```python
from build123d import *

# Parameters (mm, degrees)
SKETCH_1_W          = 270
SKETCH_1_H          = 136
EXTRUDE_1_DEPTH     = 278
SKETCH_2_W          = 266
SKETCH_2_H          = 274
CUT_EXTRUDE_1_DEPTH = 134
CUT_EXTRUDE_2_REACH = 318.438
SKETCH_3_W          = 100
SKETCH_3_H          = 40
CUT_EXTRUDE_3_REACH = 318.438
SKETCH_4_W          = 1
SKETCH_4_H          = 4


with BuildPart() as part:
    # 草图1 → 凸台-拉伸1 (new body)
    with BuildSketch(Plane(origin=(0, 0, 0), x_dir=(1, 0, 0), z_dir=(0, 1, 0))):
        Rectangle(SKETCH_1_W, SKETCH_1_H)
    extrude(amount=EXTRUDE_1_DEPTH)

    # 草图2 → 切除-拉伸1 (cut)
    with BuildSketch(Plane(origin=(0, 0, -68), x_dir=(-1, 0, 0), z_dir=(0, 0, -1))):
        with Locations((0, 139)):
            Rectangle(SKETCH_2_W, SKETCH_2_H)
    extrude(amount=-CUT_EXTRUDE_1_DEPTH, mode=Mode.SUBTRACT)

    # 草图3 → 切除-拉伸2 (cut, up to next)
    with BuildSketch(Plane(origin=(0, 278, 0), x_dir=(1, 0, 0), z_dir=(0, 1, 0)), mode=Mode.PRIVATE) as cut_extrude_2_sk1:
        with Locations((0, 48)):
            Rectangle(SKETCH_3_W, SKETCH_3_H)
    cut_extrude_2_tool1 = extrude(cut_extrude_2_sk1.sketch, amount=-CUT_EXTRUDE_2_REACH, mode=Mode.PRIVATE) & part.part
    add(cut_extrude_2_tool1.solids().sort_by_distance((0, 278, -48))[0], mode=Mode.SUBTRACT)

    # 草图4 → 切除-拉伸3 (cut, up to next)
    with BuildSketch(Plane.XZ, mode=Mode.PRIVATE) as cut_extrude_3_sk1:
        with Locations((-134.5, 42)):
            Rectangle(SKETCH_4_W, SKETCH_4_H)
    cut_extrude_3_tool1 = extrude(cut_extrude_3_sk1.sketch, amount=-CUT_EXTRUDE_3_REACH, mode=Mode.PRIVATE) & part.part
    # 草图4 → 切除-拉伸3 (cut, up to next)
    with BuildSketch(Plane.XZ, mode=Mode.PRIVATE) as cut_extrude_3_sk2:
        with Locations((-134.5, -42)):
            Rectangle(SKETCH_4_W, SKETCH_4_H)
    cut_extrude_3_tool2 = extrude(cut_extrude_3_sk2.sketch, amount=-CUT_EXTRUDE_3_REACH, mode=Mode.PRIVATE) & part.part
    # 草图4 → 切除-拉伸3 (cut, up to next)
    with BuildSketch(Plane.XZ, mode=Mode.PRIVATE) as cut_extrude_3_sk3:
        with Locations((134.5, -42)):
            Rectangle(SKETCH_4_W, SKETCH_4_H)
    cut_extrude_3_tool3 = extrude(cut_extrude_3_sk3.sketch, amount=-CUT_EXTRUDE_3_REACH, mode=Mode.PRIVATE) & part.part
    # 草图4 → 切除-拉伸3 (cut, up to next)
    with BuildSketch(Plane.XZ, mode=Mode.PRIVATE) as cut_extrude_3_sk4:
        with Locations((134.5, 42)):
            Rectangle(SKETCH_4_W, SKETCH_4_H)
    cut_extrude_3_tool4 = extrude(cut_extrude_3_sk4.sketch, amount=-CUT_EXTRUDE_3_REACH, mode=Mode.PRIVATE) & part.part
    add(cut_extrude_3_tool1.solids().sort_by_distance((-134.5, 0, 42))[0], mode=Mode.SUBTRACT)
    add(cut_extrude_3_tool2.solids().sort_by_distance((-134.5, 0, -42))[0], mode=Mode.SUBTRACT)
    add(cut_extrude_3_tool3.solids().sort_by_distance((134.5, 0, -42))[0], mode=Mode.SUBTRACT)
    add(cut_extrude_3_tool4.solids().sort_by_distance((134.5, 0, 42))[0], mode=Mode.SUBTRACT)


solid = part.part
```
Part model, mm, in its own coordinate system. A direction names the side the tool comes from. Round coordinates to 2 decimals unless told otherwise and drop trailing zeros. Loops run counter-clockwise (first coordinate to the right, second up) from the corner with the lowest first, then second, coordinate; pieces in that order, holes last. Notation, with made-up numbers: (57.25, 77.25) -> (112.25, 77.25) arc R20 cw to (112.25, 103.25) -> close; hole circle Ø2 at (18, -10.75). An arc over 180 degrees is marked (long way). Use a Markdown table: item, result.
1) Cut at D-D, the plane z = -49. List the corners of the cut face in (x, y), and give its area (3 significant figures).
The answers:
| item | result |
|---|---|
| outline | (-135, 0) -> (135, 0) -> (135, 278) -> (50, 278) -> (50, 276) -> (133, 276) -> (133, 2) -> (-133, 2) -> (-133, 276) -> (-50, 276) -> (-50, 278) -> (-135, 278) -> close |
| area | 1,980 mm2 |
2) Probe line 1 (X direction, y = 107, z = -39.5); line 2 (Y direction, x = 24, z = -24); line 3 (Z direction, x = 98, y = 109.5). List the from-to ranges inside material, lowest first. Write a range as [from, to].
The answers:
| item | result |
|---|---|
| line 1 | x = [-135, -133], [133, 135] |
| line 2 | y = [0, 2], [276, 278] |
| line 3 | z = [66, 68] |
3) Tool access for faces 4 (the flat face through (-2, 0, -1)), 5 (the flat face through (-133, 137, -2)): list every direction of +Z, -Z, +X, -X, +Y, -Y with a clear straight run to the whole face (end or side of a thin tool).
The answers:
| item | result |
|---|---|
| face 4 | +Z, -Z, +X, -X, -Y |
| face 5 | -Z |
4) Cut at A-A, the plane z = 11. List the corners of the cut face in (x, y), and give its area (3 significant figures).
The answers:
| item | result |
|---|---|
| outline | (-135, 0) -> (135, 0) -> (135, 278) -> (-135, 278) -> close; hole (-133, 2) -> (133, 2) -> (133, 276) -> (-133, 276) -> close |
| area | 2,180 mm2 |
5) Drop flat-ended pins along their axis: pin 1 Ø1.6 at (x, y) = (-17, 276.5) entering from -Z; pin 2 Ø10 at (x, y) = (54.5, 219) entering from -Z; pin 3 Ø1 at (y, z) = (277, -42) entering from -X. Give the stop position or say it passes through.
The answers:
| item | result |
|---|---|
| pin 1 | stops at z = -28 |
| pin 2 | stops at z = 66 |
| pin 3 | stops at x = -134 |
6) Pull direction X, two halves, no side cores. Call faces 1 (the flat face through (-2, 278, -1)), 2 (the flat face through (2, 141, 66)), 3 (the flat face through (-135, 137, 1)): pulls with the +X half, pulls with the -X half, needs draft (parallel to the pull), parting line crosses it, or undercut.
The answers:
| item | result |
|---|---|
| face 1 | needs draft |
| face 2 | undercut |
| face 3 | pulls with the -X half |
7) Cut at B-B, the plane x = 102.5. List the corners of the cut face in (y, z).
The answers:
| item | result |
|---|---|
| outline | (0, -68) -> (2, -68) -> (2, 66) -> (276, 66) -> (276, -68) -> (278, -68) -> (278, 68) -> (0, 68) -> close |
8) Cut at C-C, the plane y = 32. List the corners of the cut face in (x, z), and give its area (3 significant figures).
The answers:
| item | result |
|---|---|
| outline | (-135, -68) -> (-133, -68) -> (-133, 66) -> (133, 66) -> (133, -68) -> (135, -68) -> (135, -44) -> (134, -44) -> (134, -40) -> (135, -40) -> (135, 40) -> (134, 40) -> (134, 44) -> (135, 44) -> (135, 68) -> (-135, 68) -> (-135, 44) -> (-134, 44) -> (-134, 40) -> (-135, 40) -> (-135, -40) -> (-134, -40) -> (-134, -44) -> (-135, -44) -> close |
| area | 1,060 mm2 |
